Geometry check sheet. Reference: the model listing, model coordinates, mm. A direction names the side the tool comes from. Give positions to 0.01 mm unless a question says otherwise; leave off trailing zeros. Loops run counter-clockwise (first coordinate to the right, second up) from the corner with the lowest first, then second, coordinate; pieces in that order, holes last. Notation, with made-up numbers: (-10, -24.5) -> (36, -24.5) arc R18 cw to (36, 7.5) -> close; hole circle Ø6 at (18, 50). An arc over 180 degrees is marked (long way). One line per item, written item: value. Start each with the question number.
(1) Sectioned sample at B-B, the plane x = -8. Record the cut outline in (y, z).
(2) Scan lines: line 1 along Y through (x, z) = (-23.5, 3); line 2 along Z through (x, y) = (-5, 1.65); line 3 along X through (y, z) = (1.65, 2.5). Record each from-to range of solid material in increasing order. Write a range as from..to.
(3) Sectioned sample at A-A, the plane z = 1. Record the cut outline in (x, y), then the cut area to 3 significant figures.
(4) Sectioned sample at C-C, the plane y = 2.6. Record the cut outline in (x, z), then the cut area to 3 significant figures.
(5) Tool access check on faces 1 (the face through (-20.76, 1.48, -0.3)), 2 (the face through (-12, 1, 10.117)), 3 (the face through (0.723, 3.5, 2.4)), 4 (the face through (-3.614, 1.479, -0.046)). Record the directions out of +Z, -Z, +X, -X, +Y, -Y that give a thin tool (end or side, any length) a straight path to the whole face; none if there is none.
from build123d import *

# Parameters (mm, degrees)
SKETCH1_W           = 23.8
SKETCH1_H           = 18
BOSS_EXTRUDE1_DEPTH = 3
FILLET1_R           = 18.2
SKETCH2_W           = 26
SKETCH2_H           = 20
BOSS_EXTRUDE2_DEPTH = 1


with BuildPart() as part:
    # Sketch1 → Boss-Extrude1 (new body)
    with BuildSketch(Plane(origin=(0, 0, 0), x_dir=(1, 0, 0), z_dir=(0, 1, 0))):
        with Locations((-12.277059049, -1.117021277)):
            Rectangle(SKETCH1_W, SKETCH1_H)
    extrude(amount=BOSS_EXTRUDE1_DEPTH)

    # Fillet1
    # the kernel refuses this fillet: 18.2 mm, written as the material it takes off along each edge
    with BuildSketch(Plane(origin=(-24.177059049, -45.497252664, -7.882978723), x_dir=(1, 0, 0), z_dir=(0, 1, 0))) as fillet1_piece_1:
        with BuildLine():
            CenterArc((18.198901066, -18.2), FILLET1_R, 90, 89.370363377)
            Line((0, -18), (-0.363978021, -17.996))
            ThreePointArc((-0.363978021, -17.996), (-0.364, -9), (-0.364, 0))
            Line((-0.364, 0), (0, 0.364))
            Line((0, 0.364), (18.198901066, 0.364))
            Line((18.198901066, 0.364), (18.198901066, 0))
        make_face()
    extrude(amount=93.994505329, mode=Mode.SUBTRACT)
    with BuildSketch(Plane(origin=(-0.377059049, -45.497252664, -7.882978723), x_dir=(-1, 0, 0), z_dir=(0, 1, 0))) as fillet1_piece_2:
        with BuildLine():
            CenterArc((18.198901066, 18.2), FILLET1_R, 180.629636623, 89.370363377)
            Line((0, 18), (-0.363978021, 17.996))
            ThreePointArc((-0.363978021, 17.996), (-0.364, 9), (-0.364, 0))
            Line((-0.364, 0), (0, -0.364))
            Line((0, -0.364), (18.198901066, -0.364))
            Line((18.198901066, -0.364), (18.198901066, 0))
        make_face()
    extrude(amount=93.994505329, mode=Mode.SUBTRACT)

    # Sketch2 → Boss-Extrude2 (add)
    with BuildSketch(Plane(origin=(0, 3, 0), x_dir=(1, 0, 0), z_dir=(0, 1, 0))):
        with Locations((-12.277059049, -2.262026244)):
            Rectangle(SKETCH2_W, SKETCH2_H)
    extrude(amount=BOSS_EXTRUDE2_DEPTH)


solid = part.part
Calculated:
1. outline: (0, -4.49) -> (3, -4.49) -> (3, -7.74) -> (4, -7.74) -> (4, 12.26) -> (3, 12.26) -> (3, 10.12) -> (0, 10.12) -> close
2. line 1: y = 3..4
2. line 2: z = -1.8..10.12
2. line 3: x = -22.41..-2.14
3. outline: (-25.28, 3) -> (-21.61, 3) -> (-21.61, 0) -> (-2.94, 0) -> (-2.94, 3) -> (0.72, 3) -> (0.72, 4) -> (-25.28, 4) -> close
3. area: 82.0 mm2
4. outline: (-24.18, 10.12) arc R18.2 ccw to (-12.28, -6.76) arc R18.2 ccw to (-0.38, 10.12) -> close
4. area: 291 mm2
5. face 1: -Z, -X, -Y
5. face 2: +Z, +X, -X, -Y
5. face 3: +Z, -Z, +X, +Y, -Y
5. face 4: -Z, +X, -Y
